Can you work these out from the model? Positions are in its coordinate system, mm. A direction names the side the tool comes from. Coordinates: 2 decimals unless noted, no trailing zeros. Order: outer loops, then holes, each group sorted by start corner. A loop starts at its lowest first (then second) coordinate and runs counter-clockwise, first axis right, second up. Notation, with made-up numbers: (31.5, 69.25) - (46.5, 69.25) arc R19 ccw to (46.5, 87.25) - close; hole circle Ø2 at (69, 49.25). An arc over 180 degrees is marked (long way). Use a Markdown table: item, result. Add a question column.
(1) I want a section at D-D (y = 1218). List the corners of the cut face in (x, z) for me, and give its area (3 significant figures).
(2) For pin 1 Ø1.8 at (y, z) = (1216, 4) entering from +X; pin 2 Ø1.8 at (x, z) = (3432, 3) entering from +Y; pin 3 Ø3 at (x, z) = (3419, 3) entering from -Y, each with a flat end and sliding along its axis, tell me the tip position at first contact or that it passes through.
(3) I want a section at B-B (y = 1202). List the corners of the cut face in (x, z) for me, and give its area (3 significant figures).
(4) We'd pull the mould along Y, two halves only. Please class faces 1 (the flat face through (3432, 1197.661, 3)), 2 (the flat face through (3406, 1219.661, 3)), 3 (the flat face through (3418, 1219, 0)): pulls with the +Y half, pulls with the -Y half, needs draft (parallel to the pull), parting line crosses it, or undercut.
(5) I want a section at C-C (x = 3418). List the corners of the cut face in (y, z) for me.
(6) On a 3-axis mill with a long thin cutter (end or side, diameter ignored), from which of +Z, -Z, +X, -X, +Y, -Y can I reach the whole of each face in a straight line? I mean faces 4 (the flat face through (3434.744, 1201, 3)), 5 (the flat face through (3390.744, 1201, 3)), 6 (the flat face through (3413, 1203.661, 3)), 7 (the flat face through (3432, 1219.661, 3)). Say none if no direction works.
(7) If I drill on L1, parallel to Y at x = 3418.5, z = 5.75; L2, parallel to X at y = 1219.5, z = 3.7; L3, parallel to X at y = 1201, z = 4.75, over which ranges is the centre line in solid material (lowest first)? Write a range as [from, to].
```python
from build123d import *

# Parameters (mm, degrees)
MODEL_W             = 6
MODEL_H             = 6
BOSS_EXTRUDE1_DEPTH = 6


with BuildPart() as part:
    # Model → Boss-Extrude1 (new body)
    with BuildSketch(Plane.XY):
        with BuildLine():
            Line((3428.744099931, 1203.660512719), (3428.744099931, 1197.660512719))
            Line((3428.744099931, 1197.660512719), (3434.744099931, 1197.660512719))
            Line((3434.744099931, 1197.660512719), (3434.744099931, 1203.660512719))
            Line((3434.744099931, 1203.660512719), (3455.601242788, 1203.660512719))
            ThreePointArc((3455.601242788, 1203.660512719), (3418.744099931, 1240.517655576), (3381.886957074, 1203.660512719))
            Line((3381.886957074, 1203.660512719), (3390.744099931, 1203.660512719))
            Line((3390.744099931, 1203.660512719), (3390.744099931, 1197.660512719))
            Line((3390.744099931, 1197.660512719), (3396.744099931, 1197.660512719))
            Line((3396.744099931, 1197.660512719), (3396.744099931, 1203.660512719))
            Line((3396.744099931, 1203.660512719), (3428.744099931, 1203.660512719))
        make_face()
        with Locations((3431.744099931, 1216.660512719)):
            Rectangle(MODEL_W, MODEL_H, mode=Mode.SUBTRACT)
        with Locations((3405.744099931, 1216.660512719)):
            Rectangle(MODEL_W, MODEL_H, mode=Mode.SUBTRACT)
        with Locations((3418.744099931, 1222.660512719)):
            Rectangle(MODEL_W, MODEL_H, mode=Mode.SUBTRACT)
        with Locations((3418.744099931, 1210.484971552)):
            Rectangle(MODEL_W, MODEL_H, mode=Mode.SUBTRACT)
    extrude(amount=BOSS_EXTRUDE1_DEPTH)


solid = part.part
```
Answers follow:
| question | item | result |
|---|---|---|
| 1 | outline | (3384.79, 0) - (3402.74, 0) - (3402.74, 6) - (3384.79, 6) - close; (3408.74, 0) - (3428.74, 0) - (3428.74, 6) - (3408.74, 6) - close; (3434.74, 0) - (3452.7, 0) - (3452.7, 6) - (3434.74, 6) - close |
| 1 | area | 335 mm² |
| 2 | pin 1 | stops at x = 3453.78 |
| 2 | pin 2 | stops at y = 1238.38 |
| 2 | pin 3 | stops at y = 1203.66 |
| 3 | outline | (3390.74, 0) - (3396.74, 0) - (3396.74, 6) - (3390.74, 6) - close; (3428.74, 0) - (3434.74, 0) - (3434.74, 6) - (3428.74, 6) - close |
| 3 | area | 72.0 mm² |
| 4 | face 1 | pulls with the -Y half |
| 4 | face 2 | undercut |
| 4 | face 3 | needs draft |
| 5 | outline | (1203.66, 0) - (1207.48, 0) - (1207.48, 6) - (1203.66, 6) - close; (1213.48, 0) - (1219.66, 0) - (1219.66, 6) - (1213.48, 6) - close; (1225.66, 0) - (1240.51, 0) - (1240.51, 6) - (1225.66, 6) - close |
| 6 | face 4 | +Z, -Z, +X, -Y |
| 6 | face 5 | +Z, -Z, -X, -Y |
| 6 | face 6 | +Z, -Z, -Y |
| 6 | face 7 | +Z, -Z |
| 7 | L1 | y = [1203.66, 1207.48], [1213.48, 1219.66], [1225.66, 1240.52] |
| 7 | L2 | x = [3385.46, 3402.74], [3408.74, 3428.74], [3434.74, 3452.02] |
| 7 | L3 | x = [3390.74, 3396.74], [3428.74, 3434.74] |
